Source: CAD feature listing. Evaluate the final solid. Frame: model axes, mm. Face numbers are marked on the shaded views. Give positions to 0.01 mm unless a question says otherwise; leave off trailing zeros. Loops run counter-clockwise (first coordinate to the right, second up) from the corner with the lowest first, then second, coordinate; pieces in that order, holes last. Notation, with made-up numbers: (1.5, 24.25) -> (25.5, 24.25) arc R22 ccw to (25.5, 37.25) -> close; hole circle Ø1 at (-7.75, 22). An arc over 180 degrees is marked (long way). Return JSON: item names as keys, results as strings. Group by question number.
(1) Ray query, line 1 (Z direction, x = 20, y = 11.5); line 2 (Z direction, x = 20.5, y = 14.5); line 3 (Y direction, x = -6.5, z = 33). Return the intervals inside material, ascending. Write a range as from..to.
(2) Cut plane C-C on x = 0. Return loops of the section in (y, z).
(3) Cut plane B-B on y = 5. Return loops of the section in (x, z).
(4) Cut plane A-A on z = 11.5. Return loops of the section in (x, y).
(5) Pin query (flat end, axial travel): pin 1 (3 mm diameter, centred on x = -2, y = 30.5, fed in from +Z); pin 2 (6.5 mm diameter, centred on x = 20, z = 8, fed in from +Y); pin 3 (3.5 mm diameter, centred on x = 20, z = 32, fed in from -Y). Return the tip coordinate at first contact, or that it passes through.
(6) Cut plane D-D on y = 20. Return loops of the section in (x, z).
(7) Draft query along Y for the marked faces 1, 2, 3 and 4. Return one class per face: released by +Y, released by -Y, zero draft, split by the parting line, or undercut.
```python
from build123d import *

# Parameters (mm, degrees)
AUFSATZ_LINEAR_AUSTRAGEN1_DEPTH = 40
SKIZZE2_R                       = 14
SCHNITT_LINEAR_AUSTRAGEN1_DEPTH = 40
SKIZZE3_R                       = 2.1
SCHNITT_LINEAR_AUSTRAGEN2_DEPTH = 15


with BuildPart() as part:
    # Skizze1 → Aufsatz-Linear austragen1 (new body)
    with BuildSketch(Plane.XY):
        Polygon((-26, 0), (26, 0), (26, 26), (12, 40), (-12, 40), (-26, 26), align=None)
    extrude(amount=AUFSATZ_LINEAR_AUSTRAGEN1_DEPTH)

    # Skizze2 → Schnitt-Linear austragen1 (cut)
    with BuildSketch(Plane.XY.offset(40)):
        with Locations((0, 20)):
            Circle(SKIZZE2_R)
    extrude(amount=-SCHNITT_LINEAR_AUSTRAGEN1_DEPTH, mode=Mode.SUBTRACT)

    # Skizze3 → Schnitt-Linear austragen2 (cut)
    with BuildSketch(Plane.XZ):
        with Locations((-20, 32)):
            Circle(SKIZZE3_R)
        with Locations((20, 32)):
            Circle(SKIZZE3_R)
        with Locations((-20, 8)):
            Circle(SKIZZE3_R)
        with Locations((20, 8)):
            Circle(SKIZZE3_R)
    extrude(amount=-SCHNITT_LINEAR_AUSTRAGEN2_DEPTH, mode=Mode.SUBTRACT)


solid = part.part
```
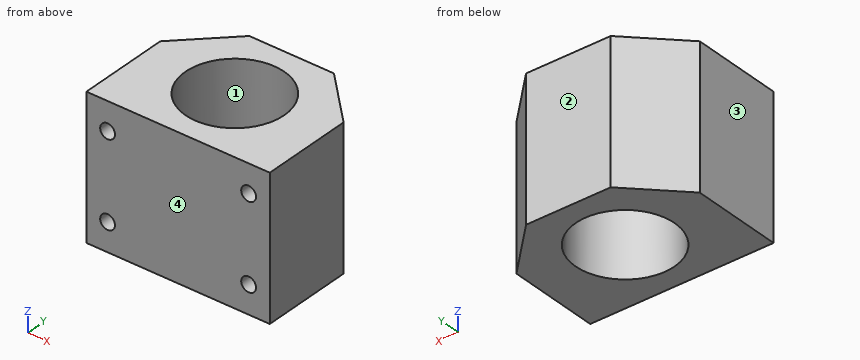
Answers:
{
 "1": {"line 1": "0..5.9, 10.1..29.9, 34.1..40", "line 2": "0..5.96, 10.04..29.96, 34.04..40", "line 3": "0..7.6, 32.4..40"},
 "2": {"outline": "(0, 0) -> (6, 0) -> (6, 40) -> (0, 40) -> close; (34, 0) -> (40, 0) -> (40, 40) -> (34, 40) -> close"},
 "3": {"outline": "(-26, 0) -> (26, 0) -> (26, 40) -> (-26, 40) -> close; hole circle Ø4.2 at (-20, 8); hole circle Ø4.2 at (-20, 32); hole circle Ø4.2 at (20, 8); hole circle Ø4.2 at (20, 32)"},
 "4": {"outline": "(-26, 0) -> (26, 0) -> (26, 26) -> (12, 40) -> (-12, 40) -> (-26, 26) -> close; hole circle Ø28 at (0, 20)"},
 "5": {"pin 1": "through", "pin 2": "y = 35.25", "pin 3": "y = 15"},
 "6": {"outline": "(-26, 0) -> (-14, 0) -> (-14, 40) -> (-26, 40) -> close; (14, 0) -> (26, 0) -> (26, 40) -> (14, 40) -> close"},
 "7": {"face 1": "undercut", "face 2": "released by +Y", "face 3": "zero draft", "face 4": "released by -Y"}
}
